Input: part model. Units: mm. Frame: model coordinates. Face numbers are marked on the shaded views. Give positions to 0.01 mm unless a question says otherwise; leave off trailing zeros. Order: outer loops, then holes, each group sorted by start corner. A loop starts at its lowest first (then second) coordinate and runs counter-clockwise, first axis right, second up. Notation, with made-up numbers: M 25,61 L 63,61 A33 ccw 63,99 Z; hole C 42.5,58.5 d3. An arc over 180 degrees is marked long. Use a Markdown table: item, result.
from build123d import *

# Parameters (mm, degrees)
SKETCH_1_W      = 50
SKETCH_1_H      = 50
SKETCH_1_R      = 1.65
SKETCH_1_R_2    = 6.25
EXTRUDE_1_DEPTH = 4


with BuildPart() as part:
    # 草图1 → 凸台-拉伸1 (new body)
    with BuildSketch(Plane.XY):
        Rectangle(SKETCH_1_W, SKETCH_1_H)
        with Locations((-20, -20)):
            Circle(SKETCH_1_R, mode=Mode.SUBTRACT)
        with Locations((-20, 20)):
            Circle(SKETCH_1_R, mode=Mode.SUBTRACT)
        with Locations((20, 20)):
            Circle(SKETCH_1_R, mode=Mode.SUBTRACT)
        with Locations((20, -20)):
            Circle(SKETCH_1_R, mode=Mode.SUBTRACT)
        Circle(SKETCH_1_R_2, mode=Mode.SUBTRACT)
    extrude(amount=EXTRUDE_1_DEPTH)


solid = part.part
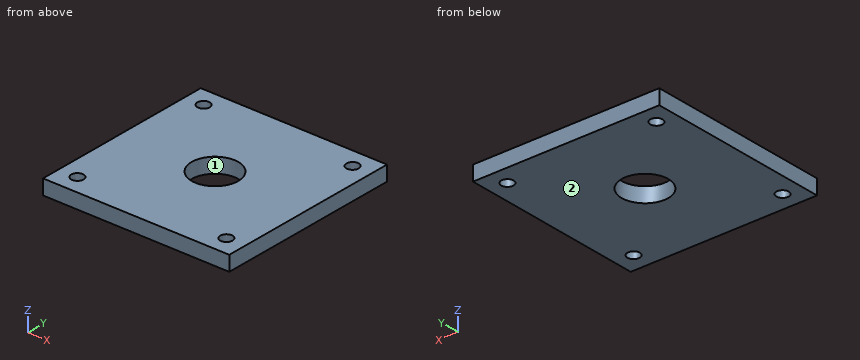
1) Cut plane A-A on y = 0. Return loops of the section in (x, z).
Response values:
| item | result |
|---|---|
| outline | M -25,0 L -6.25,0 L -6.25,4 L -25,4 Z; M 6.25,0 L 25,0 L 25,4 L 6.25,4 Z |
2) Material intervals for line 1 (Y direction, x = 20, z = 1.6); line 2 (X direction, y = 20.5, z = 0.5); line 3 (Y direction, x = 0, z = 1.85), sorted ascending. Write a range as from..to.
Response values:
| item | result |
|---|---|
| line 1 | y = -25..-21.65, -18.35..18.35, 21.65..25 |
| line 2 | x = -25..-21.57, -18.43..18.43, 21.57..25 |
| line 3 | y = -25..-6.25, 6.25..25 |
3) Mould query, pull axis X, two halves, no side actions, for the marked faces 1 and 2. Classes: released by +X, released by -X, zero draft, split by the parting line, or undercut.
Response values:
| item | result |
|---|---|
| face 1 | undercut |
| face 2 | zero draft |
4) Cut plane B-B on y = 20. Return loops of the section in (x, z), and give its area (3 significant figures).
Response values:
| item | result |
|---|---|
| outline | M -25,0 L -21.65,0 L -21.65,4 L -25,4 Z; M -18.35,0 L 18.35,0 L 18.35,4 L -18.35,4 Z; M 21.65,0 L 25,0 L 25,4 L 21.65,4 Z |
| area | 174 mm² |
5) Cut plane D-D on z = 2.5. Return loops of the section in (x, y).
Response values:
| item | result |
|---|---|
| outline | M -25,-25 L 25,-25 L 25,25 L -25,25 Z; hole C -20,-20 d3.3; hole C -20,20 d3.3; hole C 0,0 d12.5; hole C 20,-20 d3.3; hole C 20,20 d3.3 |
